```python
from build123d import *

# Parameters (mm, degrees)
BASPROSKE_W      = 18
BASPROSKE_H      = 32
TOOTHCUT_DEPTH   = 49.703182648
TEETHCUTS_COUNT  = 30
HUBNEAONESKE_R   = 24
HUBNEARONE_DEPTH = 12.0000508
BORSKE_R         = 16
BORE_DEPTH       = 30.0000508
KEYSKE_W         = 10
KEYSKE_H         = 19.3
KEYWAY_DEPTH     = 30.0000508
SMUSSO1_SIZE     = 1
RACCORDO1_R      = 1


with BuildPart() as part:
    # BasProSke → Base-Revolve (revolve)
    with BuildSketch(Plane(origin=(0, 0, 0), x_dir=(1, 0, 0), z_dir=(0, 1, 0)), mode=Mode.PRIVATE) as base_revolve_sk:
        with Locations((9, 16)):
            Rectangle(BASPROSKE_W, BASPROSKE_H)
    revolve(base_revolve_sk.sketch.rotate(Axis((-10, 0, 0), (1, 0, 0)), 180), axis=Axis((-10, 0, 0), (1, 0, 0)))

    # TooCutSke → ToothCut (cut, through all)
    with BuildSketch(Plane(origin=(0, 0, 0), x_dir=(0, 0, -1), z_dir=(1, 0, 0))):
        with BuildLine():
            ThreePointArc((0.918551563, 27.483654488), (0, 27.499), (-0.918551563, 27.483654488))
            ThreePointArc((-0.918551563, 27.483654488), (-1.617208176, 29.787801627), (-2.761784709, 31.906093311))
            ThreePointArc((-2.761784709, 31.906093311), (0, 32.0254), (2.761784709, 31.906093311))
            ThreePointArc((2.761784709, 31.906093311), (1.617208176, 29.787801627), (0.918551563, 27.483654488))
        make_face()
    toothcut = extrude(amount=TOOTHCUT_DEPTH, mode=Mode.SUBTRACT)

    # TeethCuts: ToothCut ×30 about axis
    teethcuts_axis = Axis((0, 0, 0), (1, 0, 0))
    for i in range(1, TEETHCUTS_COUNT):
        add(toothcut.rotate(teethcuts_axis, i * 360 / TEETHCUTS_COUNT), mode=Mode.SUBTRACT)

    # HubNeaOneSke → HubNearOne (add)
    with BuildSketch(Plane.ZY):
        with Locations(Location((0, 0, 0), (0, 0, 180))):
            Circle(HUBNEAONESKE_R)
    extrude(amount=HUBNEARONE_DEPTH)

    # BorSke → Bore (cut, symmetric)
    with BuildSketch(Plane(origin=(0, 0, 0), x_dir=(0, 0, -1), z_dir=(1, 0, 0))):
        with Locations(Location((0, 0, 0), (0, 0, 180))):
            Circle(BORSKE_R)
    extrude(amount=BORE_DEPTH, both=True, mode=Mode.SUBTRACT)

    # KeySke → Keyway (cut, symmetric)
    with BuildSketch(Plane(origin=(0, 0, 0), x_dir=(0, 0, -1), z_dir=(1, 0, 0))):
        with Locations((0, 9.65)):
            Rectangle(KEYSKE_W, KEYSKE_H)
    extrude(amount=KEYWAY_DEPTH, both=True, mode=Mode.SUBTRACT)

    # Smusso1
    smusso1_edges = [part.edges().sort_by_distance(p)[0] for p in [
        (18, -16, 0),
    ]]
    chamfer(smusso1_edges, length=SMUSSO1_SIZE)

    # Raccordo1
    raccordo1_edges = [part.edges().sort_by_distance(p)[0] for p in [
        (0, 0, 24),
    ]]
    fillet(raccordo1_edges, radius=RACCORDO1_R)


solid = part.part
```
The listing builds one solid part. Answer for the finished solid, in the listing's coordinates (mm). A direction names the side the tool comes from. Coordinates: 2 decimals unless noted, no trailing zeros. Write each loop counter-clockwise with the first axis right and the second up, starting at its lowest first coordinate (ties: lowest second). Pieces come first, ordered by that corner, then holes. Notation, with made-up numbers: (22, 71) - (64, 71) arc R30 cw to (64, 104) - close; hole circle Ø8 at (71.5, -27). An arc over 180 degrees is marked (long way). Return JSON: item names as keys, results as strings. Group by question number.
Q1. Flat-ended cylindrical pins translate along their axes: pin 1 Ø8 at (x, z) = (-6.5, -17.5) entering from +Y; pin 2 Ø8 at (x, z) = (-1, -2.5) entering from -Y; pin 3 Ø1 at (x, y) = (-7, 14) entering from -Z; pin 4 Ø2 at (x, y) = (10, 18) entering from -Z. Find the tip coordinate at first contact, or state that the pin passes through.
Q2. Find the intervals of material crossed by line 1 along Y through (x, z) = (-2, 0); line 2 along Z through (x, y) = (10, 0); line 3 along Y through (x, z) = (9, 0), in increasing order. Write a range as [from, to].
Q3. Which of the six approach directions +Z, -Z, +X, -X, +Y, -Y give full straight-line access (tool end or side, diameter ignored) to faces 1 (the cylindrical face through (8.87, -4.73, -29.47)), 2 (the cylindrical face through (8.874, -23.158, 18.833)), 3 (the cylindrical face through (8.874, -18.714, -23.173))?
Q4. The part is cut by section A-A on z = 0. Write down the section's boundary in (x, y), and give its area (3 significant figures).
Q5. For a pull along Y with two mould halves and no side action, classify faces 4 (the cylindrical face through (8.87, -28.82, 7.79)), 5 (the cylindrical face through (8.874, 23.158, -18.833)), 6 (the cylindrical face through (8.87, -16.31, -25)) as +Y half, -Y half, draft (parallel to the pull), parting line (faces both ways), or undercut.
Evaluation:
{
 "1": {"pin 1": "stops at y = 19.84", "pin 2": "stops at y = -31.88", "pin 3": "stops at z = -19.84", "pin 4": "stops at z = -26.24"},
 "2": {"line 1": "y = [-24, -16], [19.3, 24]", "line 2": "z = [-32, -16], [16, 32]", "line 3": "y = [-27.5, -16], [19.3, 27.5]"},
 "3": {"face 1": "-Z, +X, -X", "face 2": "+X, -X, -Y", "face 3": "+X, -X"},
 "4": {"outline": "(-12, -24) - (-1, -24) arc R1 cw to (0, -25) - (0, -27.5) - (18, -27.5) - (18, -17) - (17, -16) - (-12, -16) - close; (-12, 19.3) - (18, 19.3) - (18, 27.5) - (0, 27.5) - (0, 25) arc R1 cw to (-1, 24) - (-12, 24) - close", "area": "507 mm2"},
 "5": {"face 4": "-Y half", "face 5": "+Y half", "face 6": "undercut"}
}
